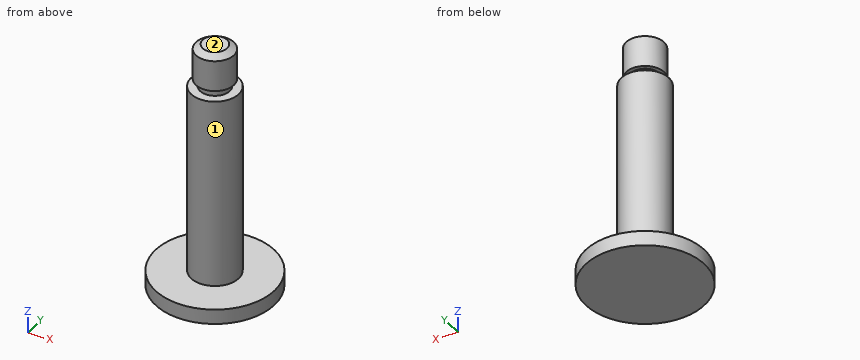
from build123d import *

# Parameters (mm, degrees)
ESQUISSE1_R        = 20
BOSS_EXTRU_1_DEPTH = 5
ESQUISSE2_R        = 8
BOSS_EXTRU_2_DEPTH = 64.25
ESQUISSE3_R        = 5
BOSS_EXTRU_3_DEPTH = 2.6
ESQUISSE4_R        = 6.4
BOSS_EXTRU_4_DEPTH = 12
CHANFREIN1_SIZE    = 1.6
CHANFREIN1_SIZE2   = 2.285036811


with BuildPart() as part:
    # Esquisse1 → Boss.-Extru.1 (new body)
    with BuildSketch(Plane.XY):
        Circle(ESQUISSE1_R)
    extrude(amount=BOSS_EXTRU_1_DEPTH)

    # Esquisse2 → Boss.-Extru.2 (add)
    with BuildSketch(Plane.XY.offset(5)):
        Circle(ESQUISSE2_R)
    extrude(amount=BOSS_EXTRU_2_DEPTH)

    # Esquisse3 → Boss.-Extru.3 (add)
    with BuildSketch(Plane.XY.offset(69.25)):
        Circle(ESQUISSE3_R)
    extrude(amount=BOSS_EXTRU_3_DEPTH)

    # Esquisse4 → Boss.-Extru.4 (add)
    with BuildSketch(Plane.XY.offset(71.85)):
        Circle(ESQUISSE4_R)
    extrude(amount=BOSS_EXTRU_4_DEPTH)

    # Chanfrein1
    chanfrein1_edges = [part.edges().sort_by_distance(p)[0] for p in [
        (-6.4, 0, 83.85),
    ]]
    chanfrein1_side = [part.faces().sort_by_distance(p)[0] for p in [
        (-6.4, 0, 77.85),
    ]]
    chamfer(chanfrein1_edges, length=CHANFREIN1_SIZE, length2=CHANFREIN1_SIZE2, reference=chanfrein1_side[0])


solid = part.part
Geometry check sheet. Reference: the model listing, model coordinates, mm. Face numbers are marked on the shaded views. A direction names the side the tool comes from. Round coordinates to 2 decimals unless told otherwise and drop trailing zeros. Order: outer loops, then holes, each group sorted by start corner. A loop starts at its lowest first (then second) coordinate and runs counter-clockwise, first axis right, second up. Notation, with made-up numbers: (-18, 16) -> (-10, 16) arc R35 ccw to (-10, 52) -> close; hole circle Ø11 at (21.5, 71.25). An arc over 180 degrees is marked (long way). Use one line per item in the form item = value.
1. Go/stop test with flat-tipped pins: pin 1 (10 mm diameter, centred on y = 11, z = 65.5, fed in from +X); pin 2 (5 mm diameter, centred on y = 8.5, z = 59, fed in from -X); pin 3 (3 mm diameter, centred on y = -1.5, z = 24, fed in from +X). Record where each tip stops, or that it passes through.
Working result:
pin_1 = 5.29
pin_2 = -5.29
pin_3 = 8
2. Cross-section at D-D, the plane x = -10.5. Enter the section's corners in (y, z).
Working result:
outline = (-17.02, 0) -> (17.02, 0) -> (17.02, 5) -> (-17.02, 5) -> close
3. Cross-section at C-C, the plane z = 15. Enter the section's corners in (x, y).
Working result:
outline = circle Ø16 at (0, 0)
4. Set-up check for the marked faces 1 and 2: record each of +Z, -Z, +X, -X, +Y, -Y from which the full face is reachable in a straight line by a thin tool's end or side.
Working result:
face_1 = +Z
face_2 = +Z, +X, -X, +Y, -Y
5. Cross-section at A-A, the plane y = 0. Enter the section's corners in (x, z), plus the area to 3 significant figures.
Working result:
outline = (-20, 0) -> (20, 0) -> (20, 5) -> (8, 5) -> (8, 69.25) -> (5, 69.25) -> (5, 71.85) -> (6.4, 71.85) -> (6.4, 82.25) -> (4.11, 83.85) -> (-4.11, 83.85) -> (-6.4, 82.25) -> (-6.4, 71.85) -> (-5, 71.85) -> (-5, 69.25) -> (-8, 69.25) -> (-8, 5) -> (-20, 5) -> close
area = 1,400 mm^2
6. Scan lines: line 1 along Z through (x, y) = (11, 2); line 2 along Y through (x, z) = (-0.5, 10); line 3 along Y through (x, z) = (5, 47) (3 decimals). Record each from-to range of solid material in increasing order. Write a range as from..to.
Working result:
line_1 = 0..5
line_2 = -7.98..7.98
line_3 = -6.245..6.245
